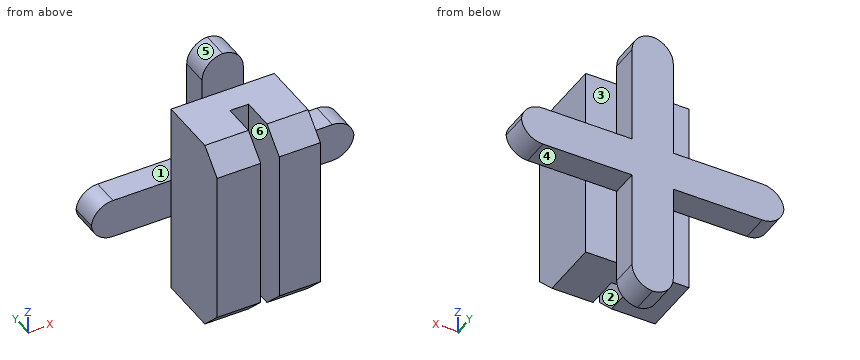
```python
from build123d import *

# Parameters (mm, degrees)
F0_W        = 19.3394050002
F0_H        = 56.1432316899
F0_W_2      = 51.9402250648
F0_H_2      = 18.5019075871
F1_DEPTH    = 12.7
F2_T1_DEPTH = 63.5
F3_W        = 48.4298244119
F3_H        = 91.9232070446
F4_DEPTH    = 12.7
F5_W        = 20.4465882853
F5_H        = 91.9232070446
F5_W_2      = 19.2932416685
F6_DEPTH    = 25.4
F7_SIZE     = 10.16


# Not quite as in the source:
# - a fillet or chamfer that OpenCascade refuses, or shapes differently, is made with other operations: its cross-section is extruded or revolved along the edge and cut away or added


with BuildPart() as f1:
    # F0 (on Front) → F1 (new body)
    with BuildSketch(Plane.XZ):
        with Locations((0, 37.3225696385)):
            Rectangle(F0_W, F0_H)
        with Locations((35.6398150325, 0)):
            Rectangle(F0_W_2, F0_H_2)
        Rectangle(F0_W, F0_H_2)
        with Locations((-35.6398150325, 0)):
            Rectangle(F0_W_2, F0_H_2)
        with Locations((0, -37.3225696385)):
            Rectangle(F0_W, F0_H)
    extrude(amount=F1_DEPTH)

    # F2: fillet of radius 10.16 on 8 edges, made by hand

    # F2_s2 → F2_t1 (cut)
    with BuildSketch(Plane.XZ.offset(-25.4)):
        with BuildLine():
            ThreePointArc((9.6697025001, 55.2341854835), (6.693907397, 62.4183903803), (-0.4902974999, 65.3941854835))
            Line((-0.4902974999, 65.3941854835), (9.6697025001, 65.3941854835))
            Line((9.6697025001, 65.3941854835), (9.6697025001, 55.2341854835))
        make_face()
        with BuildLine():
            ThreePointArc((0.4902974999, 65.3941854835), (-6.693907397, 62.4183903803), (-9.6697025001, 55.2341854835))
            Line((-9.6697025001, 55.2341854835), (-9.6697025001, 65.3941854835))
            Line((-9.6697025001, 65.3941854835), (0.4902974999, 65.3941854835))
        make_face()
        with BuildLine():
            ThreePointArc((61.6099275649, -0.9090462065), (58.6341324617, 6.2751586904), (51.4499275649, 9.2509537935))
            Line((51.4499275649, 9.2509537935), (61.6099275649, 9.2509537935))
            Line((61.6099275649, 9.2509537935), (61.6099275649, -0.9090462065))
        make_face()
        with BuildLine():
            ThreePointArc((51.4499275649, -9.2509537935), (58.6341324617, -6.2751586904), (61.6099275649, 0.9090462065))
            Line((61.6099275649, 0.9090462065), (61.6099275649, -9.2509537935))
            Line((61.6099275649, -9.2509537935), (51.4499275649, -9.2509537935))
        make_face()
        with BuildLine():
            ThreePointArc((-0.4902974999, -65.3941854835), (6.693907397, -62.4183903803), (9.6697025001, -55.2341854835))
            Line((9.6697025001, -55.2341854835), (9.6697025001, -65.3941854835))
            Line((9.6697025001, -65.3941854835), (-0.4902974999, -65.3941854835))
        make_face()
        with BuildLine():
            ThreePointArc((-51.4499275649, 9.2509537935), (-58.6341324617, 6.2751586904), (-61.6099275649, -0.9090462065))
            Line((-61.6099275649, -0.9090462065), (-61.6099275649, 9.2509537935))
            Line((-61.6099275649, 9.2509537935), (-51.4499275649, 9.2509537935))
        make_face()
        with BuildLine():
            ThreePointArc((-61.6099275649, 0.9090462065), (-58.6341324617, -6.2751586904), (-51.4499275649, -9.2509537935))
            Line((-51.4499275649, -9.2509537935), (-61.6099275649, -9.2509537935))
            Line((-61.6099275649, -9.2509537935), (-61.6099275649, 0.9090462065))
        make_face()
        with BuildLine():
            ThreePointArc((-9.6697025001, -55.2341854835), (-6.693907397, -62.4183903803), (0.4902974999, -65.3941854835))
            Line((0.4902974999, -65.3941854835), (-9.6697025001, -65.3941854835))
            Line((-9.6697025001, -65.3941854835), (-9.6697025001, -55.2341854835))
        make_face()
    extrude(amount=F2_T1_DEPTH, mode=Mode.SUBTRACT)

    # F3 (on face) → F4 (join)
    with BuildSketch(Plane.XZ.offset(12.7)):
        Rectangle(F3_W, F3_H)
    extrude(amount=F4_DEPTH)

    # F5 (on face) → F6 (join)
    with BuildSketch(Plane.XZ.offset(25.4)):
        with Locations((-13.9916180633, 0)):
            Rectangle(F5_W, F5_H)
        with Locations((14.5682913717, 0)):
            Rectangle(F5_W_2, F5_H)
    extrude(amount=F6_DEPTH)

    # F7
    f7_edges = [f1.edges().sort_by_distance(p)[0] for p in [
        (-13.991618, -50.8, 45.961604),
        (-13.991618, -50.8, -45.961604),
        (14.568291, -50.8, -45.961604),
        (14.568291, -50.8, 45.961604),
    ]]
    chamfer(f7_edges, length=F7_SIZE)


solid = f1.part
```
Model file for the job. Use its own axes, mm. Face numbers are marked on the shaded views. A direction names the side the tool comes from. Coordinates: 2 decimals unless noted, no trailing zeros. Order: outer loops, then holes, each group sorted by start corner. A loop starts at its lowest first (then second) coordinate and runs counter-clockwise, first axis right, second up. Notation, with made-up numbers: (23.25, 56) -> (35.25, 56) arc R36 ccw to (35.25, 95) -> close; hole circle Ø7 at (52, -21). An arc over 180 degrees is marked (long way). Answer as a JSON object with one key per item and string values. Group by question number.
1) Cut at C-C, the plane z = -15.5. Write the cut outline in (x, y).
2) Flat gauge pins, fed straight in: pin 1 (6 mm diameter, centred on x = -19, y = -13.5, fed in from -Z); pin 2 (10 mm diameter, centred on y = -9, z = 36, fed in from -X); pin 3 (6.5 mm diameter, centred on y = -5.5, z = -40, fed in from -X); pin 4 (5 mm diameter, centred on x = -27.5, y = -35.5, fed in from +Z). Where does each tip first touch, or does it go through?
3) Pull direction X, two halves, no side cores. Call the marked faces 4, 5 and 6: +X half, -X half, draft (parallel to the pull), parting line (faces both ways), or undercut.
4) Cut at A-A, the plane y = -10. Write the cut outline in (x, z).
5) Which spindle directions (+Z, -Z, +X, -X, +Y, -Y) get a long thin tool onto all of the face, cutting with end or side? Do the marked faces 1, 2 and 3. Say none if no direction does.
6) Cut at D-D, the plane y = -21. Write the cut outline in (x, z), then the cut area to 3 significant figures.
7) Cut at B-B, the plane x = 17. Write the cut outline in (y, z), then the cut area to 3 significant figures.
8) Drill centre lines: L1, parallel to X at y = -32.5, z = 21.5; L2, parallel to X at y = -6.5, z = -39; L3, parallel to Z at x = 4.5, y = -17.5. Where is each one in solid material? Low to high.
Check values:
{
 "1": {"outline": "(-24.21, -50.8) -> (-3.77, -50.8) -> (-3.77, -25.4) -> (4.92, -25.4) -> (4.92, -50.8) -> (24.21, -50.8) -> (24.21, -12.7) -> (9.67, -12.7) -> (9.67, 0) -> (-9.67, 0) -> (-9.67, -12.7) -> (-24.21, -12.7) -> close"},
 "2": {"pin 1": "stops at z = -45.96", "pin 2": "stops at x = -24.21", "pin 3": "stops at x = -9.67", "pin 4": "passes through"},
 "3": {"face 4": "draft", "face 5": "-X half", "face 6": "undercut"},
 "4": {"outline": "(-61.57, 0) arc R10.16 ccw to (-51.45, -9.25) -> (-9.67, -9.25) -> (-9.67, -55.23) arc R10.16 ccw to (0, -65.38) arc R10.16 ccw to (9.67, -55.23) -> (9.67, -9.25) -> (51.45, -9.25) arc R10.16 ccw to (61.57, 0) arc R10.16 ccw to (51.45, 9.25) -> (9.67, 9.25) -> (9.67, 55.23) arc R10.16 ccw to (0, 65.38) arc R10.16 ccw to (-9.67, 55.23) -> (-9.67, 9.25) -> (-51.45, 9.25) arc R10.16 ccw to start"},
 "5": {"face 1": "+Z, -X, +Y", "face 2": "+Z, -Z, -Y", "face 3": "+Z, +X, +Y"},
 "6": {"outline": "(-24.21, -45.96) -> (24.21, -45.96) -> (24.21, 45.96) -> (-24.21, 45.96) -> close", "area": "4,450 mm²"},
 "7": {"outline": "(-50.8, -35.8) -> (-40.64, -45.96) -> (-12.7, -45.96) -> (-12.7, -9.25) -> (0, -9.25) -> (0, 9.25) -> (-12.7, 9.25) -> (-12.7, 45.96) -> (-40.64, 45.96) -> (-50.8, 35.8) -> close", "area": "3,630 mm²"},
 "8": {"L1": "x = -24.21 to -3.77, 4.92 to 24.21", "L2": "x = -9.67 to 9.67", "L3": "z = -45.96 to 45.96"}
}
